Build history of the part. All positions in model axes, mm. Round coordinates to 2 decimals unless told otherwise and drop trailing zeros. Loops run counter-clockwise (first coordinate to the right, second up) from the corner with the lowest first, then second, coordinate; pieces in that order, holes last. Notation, with made-up numbers: (-19, 11.25) - (38, 11.25) arc R4 ccw to (38, 16.25) - close; hole circle Ø5 at (-1, -17). An arc over 180 degrees is marked (long way). Put each result on its own line as item: value. Start each with the question number.
from build123d import *


with BuildPart() as part:
    # Sketch1 → Revolve1 (revolve)
    with BuildSketch(Plane.XY, mode=Mode.PRIVATE) as revolve1_sk:
        with BuildLine():
            Line((6.7, -2.5), (6.7, 2.5))
            Line((6.7, 2.5), (7.7, 2.5))
            Line((7.7, 2.5), (7.7, 0.75))
            ThreePointArc((7.7, 0.75), (6.95, 0), (7.7, -0.75))
            Line((7.7, -0.75), (7.7, -2.5))
            Line((7.7, -2.5), (6.7, -2.5))
        make_face()
    revolve(revolve1_sk.sketch.rotate(Axis((0, 0, 0), (0, 1, 0)), 90), axis=Axis((0, 0, 0), (0, 1, 0)))

    # Chamfer1
    # the kernel refuses this chamfer: 0.5 mm, written as the material it takes off along each edge
    with BuildSketch(Plane(origin=(0, -0.75, 0), x_dir=(0, 0, -1), z_dir=(1, 0, 0))) as chamfer1_piece_1:
        with BuildLine():
            Line((7.389045549, 0.079346846), (7.710954451, -0.412377124))
            Line((7.710954451, -0.412377124), (7.720954451, -0.412377124))
            ThreePointArc((7.720954451, -0.412377124), (7.71, -0.206188562), (7.71, 0))
            Line((7.71, 0), (7.7, 0.01))
            ThreePointArc((7.7, 0.01), (7.54177371, 0.027113812), (7.393045549, 0.088511998))
            Line((7.393045549, 0.088511998), (7.389045549, 0.079346846))
        make_face()
    revolve(axis=Axis((0, -0.75, 0), (0, 1, 0)), mode=Mode.SUBTRACT)
    with BuildSketch(Plane(origin=(0, 0.75, 0), x_dir=(0, 0, -1), z_dir=(1, 0, 0))) as chamfer1_piece_2:
        with BuildLine():
            Line((7.710954451, 0.412377124), (7.389045549, -0.079346846))
            Line((7.389045549, -0.079346846), (7.393045549, -0.088511998))
            ThreePointArc((7.393045549, -0.088511998), (7.54177371, -0.027113812), (7.7, -0.01))
            Line((7.7, -0.01), (7.71, 0))
            ThreePointArc((7.71, 0), (7.71, 0.206188562), (7.720954451, 0.412377124))
            Line((7.720954451, 0.412377124), (7.710954451, 0.412377124))
        make_face()
    revolve(axis=Axis((0, 0.75, 0), (0, 1, 0)), mode=Mode.SUBTRACT)


solid = part.part
Item 1: Drill centre lines: probe 1 along Z at (x, y) = (-1, 0.2); probe 2 along Z at (x, y) = (-3.25, 2.2); probe 3 along X at (y, z) = (-0.05, -1). Where is each one in solid material? Low to high. Write a range as [from, to].
Item 2: Slice it at D-D (y = 0.2). Give the cut face in (x, z).
Item 3: Slice it at A-A (z = 0). Give the cut face in (x, y), plus the area to 3 significant figures.
Item 4: Slice it at B-B (x = 0). Give the cut face in (y, z).
Item 5: Drop flat-ended pins along their axis: pin 1 Ø2 at (x, y) = (-1.5, -1.5) entering from +Z; pin 2 Ø2 at (x, y) = (-5.5, -0.5) entering from -Z; pin 3 Ø1 at (y, z) = (2, -1.5) entering from +X. Give the stop position or say it passes through.
Item 6: Slice it at C-C (y = 1.95). Give the cut face in (x, z).
Computed values:
1. probe 1: z = [-6.91, -6.62], [6.62, 6.91]
1. probe 2: z = [-6.98, -5.86], [5.86, 6.98]
1. probe 3: x = [-6.88, -6.62], [6.62, 6.88]
2. outline: circle Ø13.95 at (0, 0); hole circle Ø13.4 at (0, 0)
3. outline: (-7.7, -2.5) - (-6.7, -2.5) - (-6.7, 2.5) - (-7.7, 2.5) - (-7.7, 1.15) - (-7.4, 0.69) arc R0.75 cw to (-7.4, -0.69) - (-7.7, -1.15) - close; (6.7, -2.5) - (7.7, -2.5) - (7.7, -1.15) - (7.4, -0.69) arc R0.75 cw to (7.4, 0.69) - (7.7, 1.15) - (7.7, 2.5) - (6.7, 2.5) - close
3. area: 8.01 mm^2
4. outline: (-2.5, -7.7) - (-1.15, -7.7) - (-0.69, -7.4) arc R0.75 cw to (0.69, -7.4) - (1.15, -7.7) - (2.5, -7.7) - (2.5, -6.7) - (-2.5, -6.7) - close; (-2.5, 6.7) - (2.5, 6.7) - (2.5, 7.7) - (1.15, 7.7) - (0.69, 7.4) arc R0.75 cw to (-0.69, 7.4) - (-1.15, 7.7) - (-2.5, 7.7) - close
5. pin 1: stops at z = 7.68
5. pin 2: stops at z = -6.07
5. pin 3: stops at x = 7.63
6. outline: circle Ø15.4 at (0, 0); hole circle Ø13.4 at (0, 0)
